Could you check a few things on this model? Use its own coordinates, in mm. A direction names the side the tool comes from. Give positions to 0.01 mm unless a question says otherwise; leave off trailing zeros. Loops run counter-clockwise (first coordinate to the right, second up) from the corner with the lowest first, then second, coordinate; pieces in that order, holes last. Notation, with made-up numbers: (41, -2) - (74, -2) arc R24 cw to (74, 12) - close; hole circle Ø7 at (3, -34.75). An arc over 180 degrees is marked (long way). Answer in a Markdown table with one row per item. Add a question column.
Autodesk Fusion 360 part; units mm, degrees
sketch "Sketch1" plane through (0, 0, 0) normal (0, 0, 1) x (1, 0, 0)
  line L0 (0, 0) -> (-56, 0)
  line L1 (-56, 0) -> (-56, 35)
  line L2 (0, 35) -> (0, 0)
  line L3 (-56, 0) -> (-28, 0)
  circle A0 centre (-28, 35) radius 10
  line L4 (-28, 0) -> (-4, 0)
  line L5 (-28, 35) -> (0, 35) construction
  line L6 (-28, 35) -> (-28, 0) construction
  line L7 (-4, 0) -> (-4, 35) construction
  line L8 (0, 35) -> (0, 32)
  line L9 (0, 32) -> (-4, 32)
  line L10 (-4, 32) -> (-4, 38)
  line L11 (-4, 38) -> (-0.1612, 38)
  line L12 (0, 35) -> (0, 32)
  line L13 (-28, 35) -> (-14, 59.2487) construction
  line L14 (-28, 35) -> (-42, 59.2487) construction
  line L15 (-28, 35) -> (-56, 35) construction
  line L16 (-18.5981, 57.2846) -> (-16.6787, 60.6091)
  line L17 (-11.4825, 57.6091) -> (-13.4019, 54.2846)
  line L18 (-13.4019, 54.2846) -> (-18.5981, 57.2846)
  line L19 (-42.5981, 54.2846) -> (-44.5175, 57.6091)
  line L20 (-39.3213, 60.6091) -> (-37.4019, 57.2846)
  line L21 (-37.4019, 57.2846) -> (-42.5981, 54.2846)
  line L22 (-52, 32) -> (-55.8388, 32)
  line L23 (-55.8388, 38) -> (-52, 38)
  line L24 (-52, 38) -> (-52, 32)
  line L25 (-44.5981, 12.2513) -> (-44.5175, 12.3909)
  arc A1 (-0.1612, 32) -> (-42, 59.2487) centre (-28, 35) ccw
  line L26 (-16.5981, 9.2513) -> (-16.6787, 9.3909)
  arc A2 (0, 35) -> (-11.4825, 57.6091) centre (-28, 35) ccw
  arc A3 (-14, 59.2487) -> (-56, 35) centre (-28, 35) ccw
  arc A4 (-56, 35) -> (-55.8388, 32) centre (-28, 35) ccw
  arc A5 (-42, 59.2487) -> (-55.8388, 32) centre (-28, 35) ccw
  arc A6 (-14, 59.2487) -> (-55.8388, 32) centre (-28, 35) ccw
  arc A7 (-0.1612, 32) -> (0, 35) centre (-28, 35) ccw
  arc A8 (-0.1612, 32) -> (-14, 59.2487) centre (-28, 35) ccw
  circle A9 centre (-28, 35) radius 15
  dimension "d1" = 56
  dimension "d2" = 35
  dimension "d3" = 20
  dimension "d4" = 24
  dimension "d5" = 3
  dimension "d7" = 60
  dimension "d8" = 60
  dimension "d13" = 30
extrude "Extrude1" add sketch "Sketch1" against normal blind 108 contours L0 L1 L2 L3 L4 L9 L10 L11 L16 L17 L18 L19 L20 L21 L22 L23 L24 A1 A2 A3 A4 A5 A6 A8
sketch "Sketch2" plane through (0, 0, 0) normal (1, 0, 0) x (0, 0, -1)
  line L0 (0, 32) -> (0, 0)
  line L1 (0, 0) -> (108, 0)
  line L2 (108, 0) -> (108, 32)
  line L3 (108, 32) -> (0, 32)
  line L4 (108, 0) -> (108, 56)
  line L5 (108, 56) -> (81.4419, 10)
  line L6 (108, 0) -> (108, 10)
  line L7 (108, 10) -> (81.4419, 10)
  dimension "d16" = 56
  dimension "d17" = 30
  dimension "d18" = 10
extrude "Extrude2" cut sketch "Sketch2" against normal blind 130 contours L3 L4 L5 | L2 L3 L4 L5 L7
sketch "Sketch3" plane through (0, 0, 0) normal (1, 0, 0) x (0, 0, -1)
  line L0 (81.4419, 10) -> (94.1436, 32)
  line L1 (94.1436, 32) -> (0, 32)
  line L2 (0, 32) -> (0, 0)
  line L3 (0, 0) -> (108, 0)
  line L4 (108, 0) -> (108, 10)
  line L5 (108, 10) -> (81.4419, 10)
  line L6 (81.4419, 10) -> (81.4419, 32)
  line L7 (81.4419, 32) -> (94.1436, 32)
  line L8 (94.1436, 32) -> (81.4419, 10)
extrude "Extrude3" cut sketch "Sketch3" against normal blind 140 contours L0 L1 L6 L7 L8
sketch "Sketch4" plane through (0, 0, 0) normal (0, 0, 1) x (1, 0, 0)
  circle A0 centre (-28, 35) radius 15
  line L0 (-56, 0) -> (0, 0)
  line L1 (0, 0) -> (0, 32)
  line L2 (0, 32) -> (-4, 32)
  line L3 (-4, 32) -> (-4, 38)
  line L4 (-4, 38) -> (-0.1612, 38)
  arc A1 (-0.1612, 38) -> (-11.4825, 57.6091) centre (-28, 35) ccw
  line L5 (-11.4825, 57.6091) -> (-13.4019, 54.2846)
  line L6 (-13.4019, 54.2846) -> (-18.5981, 57.2846)
  line L7 (-18.5981, 57.2846) -> (-16.6787, 60.6091)
  arc A2 (-16.6787, 60.6091) -> (-39.3213, 60.6091) centre (-28, 35) ccw
  line L8 (-39.3213, 60.6091) -> (-37.4019, 57.2846)
  line L9 (-37.4019, 57.2846) -> (-42.5981, 54.2846)
  line L10 (-42.5981, 54.2846) -> (-44.5175, 57.6091)
  arc A3 (-44.5175, 57.6091) -> (-55.8388, 38) centre (-28, 35) ccw
  line L11 (-55.8388, 38) -> (-52, 38)
  line L12 (-52, 38) -> (-52, 32)
  line L13 (-52, 32) -> (-55.8388, 32)
  arc A4 (-56, 35) -> (-55.8388, 32) centre (-28, 35) ccw
  line L14 (-56, 35) -> (-56, 0)
  circle A5 centre (-28, 35) radius 10
  dimension "d23" = 20
extrude "Extrude4" add sketch "Sketch4" against normal blind 5 contours A0
(1) For pin 1 Ø6 at (x, y) = (-46, 45.5) entering from -Z; pin 2 Ø12 at (x, y) = (-47, 18) entering from -Z; pin 3 Ø4 at (x, y) = (-46, 44.5) entering from -Z; pin 4 Ø6 at (x, y) = (-48.5, 48) entering from +Z, each with a flat end and sliding along its axis, tell me the tip position at first contact or that it passes through.
(2) We'd pull the mould along X, two halves only. Please class faces 1 (the flat face through (-2, 32, -40)), 2 (the flat face through (-56, 17, -41)), 3 (the cylindrical face through (-23.386, 26.128, -2.465)): pulls with the +X half, pulls with the -X half, needs draft (parallel to the pull), parting line crosses it, or undercut.
(3) I want a section at A-A on x = -28. Please give me the cut outline in (y, z), then the cut area to 3 significant figures.
(4) On a 3-axis mill with a long thin cutter (end or side, diameter ignored), from which of +Z, -Z, +X, -X, +Y, -Y can I reach the whole of each face in a straight line? I mean faces 4 (the flat face through (-39.96, 55.81, -53.24)), 5 (the flat face through (-4, 35, -48)), 6 (the cylindrical face through (-29.953, 49.872, -54.082)), 7 (the flat face through (-12.43, 55.97, -53.24)), 8 (the flat face through (-28, 18, -81.442)). Say none if no direction works.
(5) I want a section at B-B on y = 28.5. Please give me the cut outline in (x, z), then the cut area to 3 significant figures.
(6) I want a section at D-D on y = 17. Please give me the cut outline in (x, z), then the cut area to 3 significant figures.
(7) I want a section at C-C on z = -87. Please give me the cut outline in (x, y).
(8) Please list where these lines run through material, in increasing order: line 1 (Y direction, x = -28, z = -24); line 2 (Y direction, x = -28, z = -83); line 3 (Z direction, x = -29.5, y = 15).
Reported:
| question | item | result |
|---|---|---|
| 1 | pin 1 | z = -103.67 |
| 1 | pin 2 | z = -81.44 |
| 1 | pin 3 | z = -102.52 |
| 1 | pin 4 | z = 0 |
| 2 | face 1 | needs draft |
| 2 | face 2 | pulls with the -X half |
| 2 | face 3 | undercut |
| 3 | outline | (0, -108) - (10, -108) - (10, -81.44) - (20, -81.44) - (20, -5) - (25, -5) - (25, 0) - (0, 0) - close; (45, -5) - (50, -5) - (50, -104.54) - (56, -108) - (63, -108) - (63, 0) - (45, 0) - close |
| 3 | area | 3,340 mm² |
| 4 | face 4 | +Z, -Z |
| 4 | face 5 | +Z, -Z, +X |
| 4 | face 6 | -Z |
| 4 | face 7 | +Z, -Z, +Y |
| 4 | face 8 | -Z, +X, -X |
| 5 | outline | (-56, -81.44) - (-41.52, -81.44) - (-41.52, -5) - (-35.6, -5) - (-35.6, 0) - (-56, 0) - close; (-20.4, -5) - (-14.48, -5) - (-14.48, -81.44) - (0, -81.44) - (0, 0) - (-20.4, 0) - close |
| 5 | area | 2,420 mm² |
| 6 | outline | (-56, -81.44) - (0, -81.44) - (0, 0) - (-56, 0) - close |
| 6 | area | 4,560 mm² |
| 7 | outline | (-56, 0) - (0, 0) - (0, 10) - (-56, 10) - close; (-56, 32) - (-55.84, 32) arc R28 cw to (-56, 35) - close; (-55.84, 38) - (-52, 38) - (-52, 32) - (-42.7, 32) arc R15 cw (long way) to (-13.3, 32) - (-4, 32) - (-4, 38) - (-0.16, 38) arc R28 ccw to (-11.48, 57.61) - (-13.4, 54.28) - (-18.6, 57.28) - (-16.68, 60.61) arc R28 ccw to (-39.32, 60.61) - (-37.4, 57.28) - (-42.6, 54.28) - (-44.52, 57.61) arc R28 ccw to start |
| 8 | line 1 | 0 to 20, 50 to 63 |
| 8 | line 2 | 0 to 10, 50 to 63 |
| 8 | line 3 | -81.44 to 0 |
